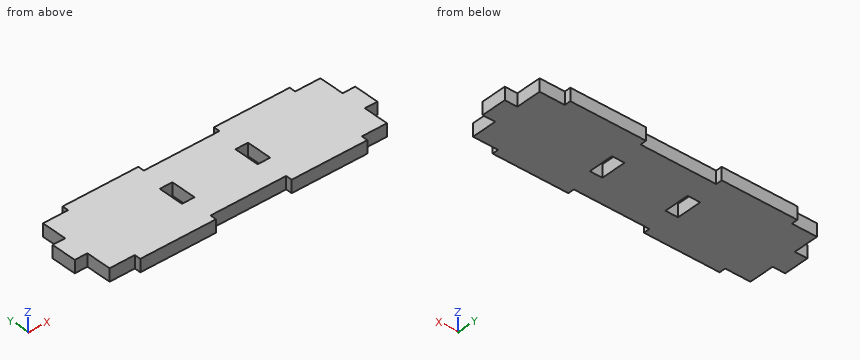
```python
from build123d import *

# Parameters (mm, degrees)
SKETCH1_W           = 304.8
SKETCH1_H           = 76.2
BOSS_EXTRUDE1_DEPTH = 12.7
SKETCH2_W           = 76.2
SKETCH2_H           = 6.35
BOSS_EXTRUDE2_DEPTH = 12.7
SKETCH3_W           = 12.7
SKETCH3_H           = 25.4
CUT_EXTRUDE1_DEPTH  = 160.257189791


with BuildPart() as part:
    # Sketch1 → Boss-Extrude1 (new body)
    with BuildSketch(Plane.XY):
        Rectangle(SKETCH1_W, SKETCH1_H)
    extrude(amount=BOSS_EXTRUDE1_DEPTH)

    # Sketch2 → Boss-Extrude2 (add)
    with BuildSketch(Plane.XY.offset(12.7)):
        with Locations((-76.2, -41.275)):
            Rectangle(SKETCH2_W, SKETCH2_H)
        with Locations((76.2, -41.275)):
            Rectangle(SKETCH2_W, SKETCH2_H)
        with Locations((76.2, 41.275)):
            Rectangle(SKETCH2_W, SKETCH2_H)
        with Locations((-76.2, 41.275)):
            Rectangle(SKETCH2_W, SKETCH2_H)
    extrude(amount=-BOSS_EXTRUDE2_DEPTH)

    # Sketch3 → Cut-Extrude1 (cut, through all)
    with BuildSketch(Plane.XY.offset(12.7)):
        with Locations((-146.05, -25.4)):
            Rectangle(SKETCH3_W, SKETCH3_H)
        with Locations((-146.05, 25.4)):
            Rectangle(SKETCH3_W, SKETCH3_H)
        with Locations((146.05, 25.4)):
            Rectangle(SKETCH3_W, SKETCH3_H)
        with Locations((146.05, -25.4)):
            Rectangle(SKETCH3_W, SKETCH3_H)
        with Locations((38.1, 0)):
            Rectangle(SKETCH3_W, SKETCH3_H)
        with Locations((-38.1, 0)):
            Rectangle(SKETCH3_W, SKETCH3_H)
    extrude(amount=-CUT_EXTRUDE1_DEPTH, mode=Mode.SUBTRACT)


solid = part.part
```
Verification items for the finished model (mm, model axes). Give positions to 0.01 mm unless a question says otherwise; leave off trailing zeros. Loops run counter-clockwise (first coordinate to the right, second up) from the corner with the lowest first, then second, coordinate; pieces in that order, holes last.
1. Section check A-A, the plane y = 6.5. Enter the section's corners in (x, z).
2. Section check B-B, the plane z = 4.5. Count the separate pieces of the cut face and the enclosed holes in it, then the cut area to 3 significant figures.
3. Section check D-D, the plane y = 21. Enter the section's corners in (x, z).
4. Thickness scan on line 1 (X direction, y = 3, z = 11.5); line 2 (X direction, y = -13, z = 4.5); line 3 (Y direction, x = -17, z = 0.75). Record the ranges inside material, lowest first.
5. Go/stop test with flat-tipped pins: pin 1 Ø1.9 at (y, z) = (42, 5.5) entering from -X; pin 2 Ø6.5 at (y, z) = (31.5, 7) entering from -X; pin 3 Ø1.9 at (y, z) = (-42.5, 6.5) entering from +X. Record where each tip stops, or that it passes through.
6. Section check C-C, the plane x = 121. Enter the section's corners in (y, z), then the cut area to 3 significant figures.
Geometry says:
1. outline: (-152.4, 0) - (-44.45, 0) - (-44.45, 12.7) - (-152.4, 12.7) - close; (-31.75, 0) - (31.75, 0) - (31.75, 12.7) - (-31.75, 12.7) - close; (44.45, 0) - (152.4, 0) - (152.4, 12.7) - (44.45, 12.7) - close
2. separate pieces: 1
2. enclosed holes: 2
2. area: 23,200 mm2
3. outline: (-139.7, 0) - (139.7, 0) - (139.7, 12.7) - (-139.7, 12.7) - close
4. line 1: x = -152.4 to -44.45, -31.75 to 31.75, 44.45 to 152.4
4. line 2: x = -139.7 to 139.7
4. line 3: y = -38.1 to 38.1
5. pin 1: stops at x = -114.3
5. pin 2: stops at x = -139.7
5. pin 3: stops at x = 114.3
6. outline: (-38.1, 0) - (38.1, 0) - (38.1, 12.7) - (-38.1, 12.7) - close
6. area: 968 mm2
